Check sheet for the drawn part. Datum: minimum x, y, z corner. Units: mm. A direction names the side the tool comes from. Give positions to 0.01 mm unless a question says otherwise; leave off trailing zeros. Order: outer loops, then holes, each group sorted by start corner. A loop starts at its lowest first (then second) coordinate and runs counter-clockwise, first axis right, second up.
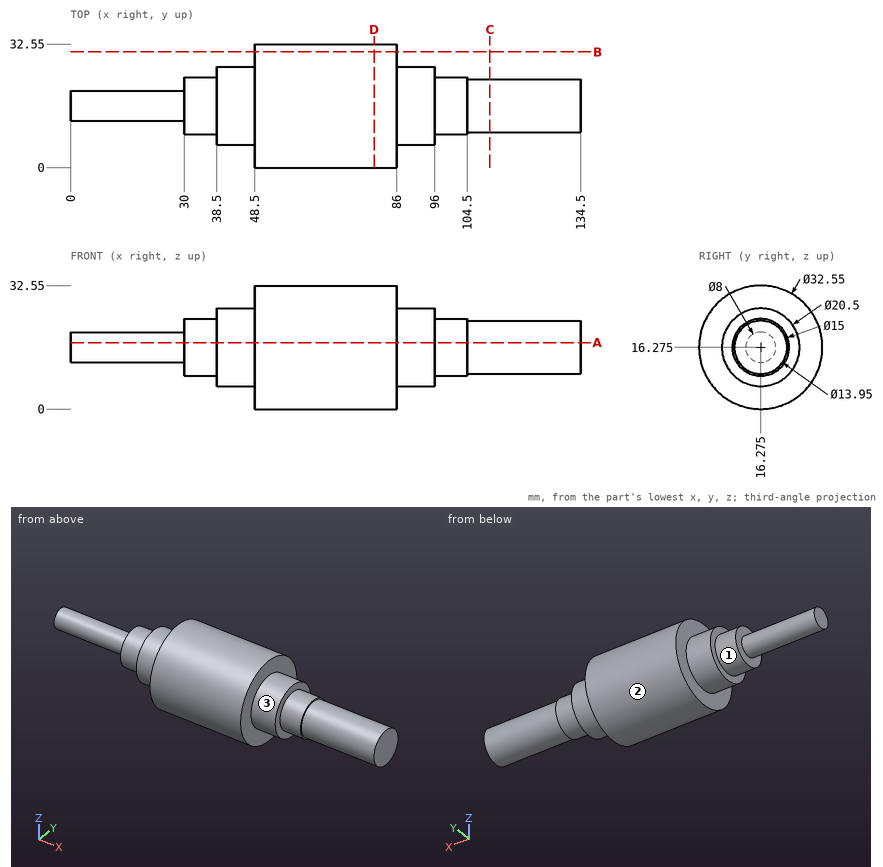
Item 1: Gauge pin test, flat ends, axial feed: pin 1 (1.5 mm diameter, centred on x = 34.5, y = 19.5, fed in from +Z); pin 2 (1 mm diameter, centred on x = 50, z = 14, fed in from +Y); pin 3 (5 mm diameter, centred on x = 39, z = 13.5, fed in from +Y). Record the tip position at first contact, or that the pin passes through.
Reported:
pin 1: stops at z = 23.35
pin 2: stops at y = 32.45
pin 3: stops at y = 26.52
Item 2: Sectioned sample at C-C (x = 110.5). Enter the section's corners in (y, z) (3 decimals).
Reported:
outline: circle Ø13.95 at (16.275, 16.275)
Item 3: Set-up check for the marked faces 1, 2 and 3: record each of +Z, -Z, +X, -X, +Y, -Y from which the full face is reachable in a straight line by a thin tool's end or side.
Reported:
face 1: -X
face 2: +X, -X
face 3: +X
Item 4: Sectioned sample at D-D (x = 80). Enter the section's corners in (y, z) (3 decimals), and give its area (3 significant figures).
Reported:
outline: circle Ø32.55 at (16.275, 16.275)
area: 832 mm2
Item 5: Sectioned sample at A-A (z = 17.5). Enter the section's corners in (x, y).
Reported:
outline: (0, 12.47) - (30, 12.47) - (30, 8.88) - (38.5, 8.88) - (38.5, 6.1) - (48.5, 6.1) - (48.5, 0.05) - (86, 0.05) - (86, 6.1) - (96, 6.1) - (96, 8.88) - (104.5, 8.88) - (104.5, 9.41) - (134.5, 9.41) - (134.5, 23.14) - (104.5, 23.14) - (104.5, 23.67) - (96, 23.67) - (96, 26.45) - (86, 26.45) - (86, 32.5) - (48.5, 32.5) - (48.5, 26.45) - (38.5, 26.45) - (38.5, 23.67) - (30, 23.67) - (30, 20.08) - (0, 20.08) - close
Item 6: Scan lines: L1, parallel to Z at x = 121, y = 22; L2, parallel to X at y = 26, z = 25; L3, parallel to X at y = 6.5, z = 16. Record each from-to range of solid material in increasing order.
Reported:
L1: z = 12.29 to 20.26
L2: x = 48.5 to 86
L3: x = 38.5 to 96
Item 7: Sectioned sample at B-B (y = 30.5). Enter the section's corners in (x, z), and give its area (3 significant figures).
Reported:
outline: (48.5, 8.37) - (86, 8.37) - (86, 24.18) - (48.5, 24.18) - close
area: 593 mm2
